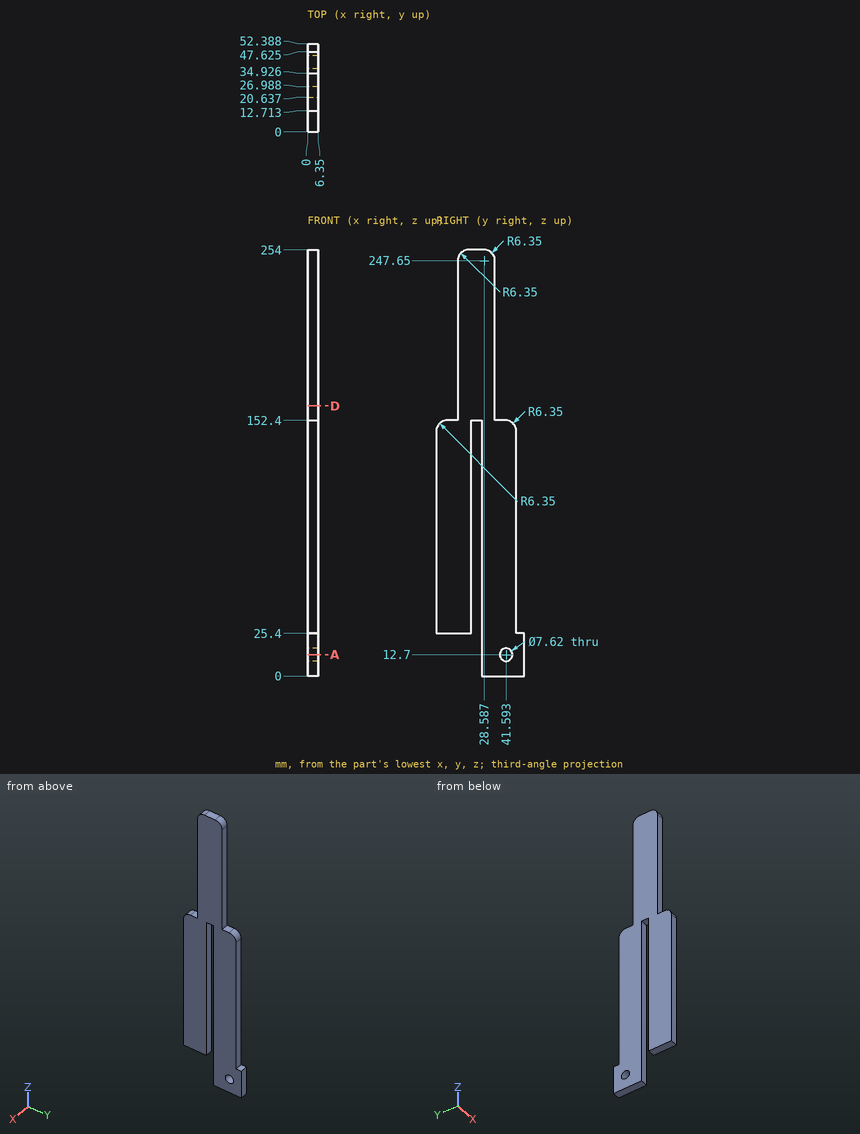
Can you work these out from the drawing? Everything is in mm from the part's minimum corner. Round coordinates to 2 decimals unless told otherwise and drop trailing zeros. Write each loop counter-clockwise with the first axis right and the second up, starting at its lowest first coordinate (ties: lowest second). Pieces come first, ordered by that corner, then holes.
1. Will these pins go through, and if not, where does the flat tip stop? pin 1 Ø2.5 at (x, y) = (2, 50.5) entering from +Z; pin 2 Ø1.9 at (x, y) = (4, 10.5) entering from +Z; pin 3 Ø1 at (x, y) = (1, 18) entering from -Z.
2. Suppose I cut it at D-D (z = 161). List the corners of the cut face in (x, y) for me, and give its area (3 significant figures).
3. I need wall thicknesses on L1, parallel to Y at x = 3.5, z = 27 (1 decimal); L2, parallel to Z at x = 5.75, y = 10.5; L3, parallel to Y at x = 1, z = 211.5. Which ranges of each line are inside material? Lowest first, please.
4. Suppose I cut it at A-A (z = 12.7). List the corners of the cut face in (x, y) for me, and give its area (3 significant figures).
Answer sheet:
1. pin 1: stops at z = 25.4
1. pin 2: stops at z = 152.4
1. pin 3: stops at z = 25.4
2. outline: (0, 12.71) - (6.35, 12.71) - (6.35, 34.93) - (0, 34.93) - close
2. area: 141 mm2
3. L1: y = 0 to 20.6, 27 to 47.6
3. L2: z = 25.4 to 152.4
3. L3: y = 12.71 to 34.93
4. outline: (0, 26.99) - (6.35, 26.99) - (6.35, 37.78) - (0, 37.78) - close; (0, 45.4) - (6.35, 45.4) - (6.35, 52.39) - (0, 52.39) - close
4. area: 113 mm2
